Check sheet for the modelled part. Datum: model origin and axes. Units: mm. A direction names the side the tool comes from. Round coordinates to 2 decimals unless told otherwise and drop trailing zeros. Loops run counter-clockwise (first coordinate to the right, second up) from the corner with the lowest first, then second, coordinate; pieces in that order, holes last. Notation, with made-up numbers: (53.5, -26.5) - (62.5, -26.5) arc R11 cw to (62.5, -5.5) - close; hole circle Ø9 at (3, -30.75). An arc over 180 degrees is marked (long way). Put each result on its own line as item: value. Start each with the question number.
Item 1: Section check A-A, the plane x = 0. Record the cut outline in (y, z), and give its area (3 significant figures).
Item 2: Section check D-D, the plane z = -2.5. Record the cut outline in (x, y), and give its area (3 significant figures).
Item 3: Gauge pin test, flat ends, axial feed: pin 1 Ø3 at (y, z) = (3, -1) entering from +X; pin 2 Ø4 at (x, z) = (-5, -5.5) entering from +Y; pin 3 Ø3 at (y, z) = (3.5, 4) entering from -X; pin 4 Ø3 at (y, z) = (10, 0.5) entering from -X. Record the tip position at first contact, or that the pin passes through.
Item 4: Material ranges on line 1 along X through (y, z) = (4.5, 0); line 2 along Y through (x, z) = (-2.5, -4), recorded low to high.
Item 5: Section check B-B, the plane z = 0. Record the cut outline in (x, y), and give its area (3 significant figures).
Item 6: Draft check along X on faces 5 (the cylindrical face through (-3.32, 6.16, -0.74)), 6 (the cylindrical face through (-6.834, 1.972, -1.517)), 7 (the flat face through (0, 12.148, 4)). Enter one of: pulls with the +X half, pulls with the -X half, needs draft (parallel to the pull), parting line crosses it, or undercut.
Item 7: Section check C-C, the plane y = 1. Record the cut outline in (x, z), and give its area (3 significant figures).
Item 8: Tool access check on faces 1 (the flat face through (2, 0, 3)), 2 (the cylindrical face through (0, 8, -5)), 3 (the flat face through (-4.5, 13.6, -1.709)), 4 (the flat face through (-4.5, 13.6, 1.709)). Record the directions out of +Z, -Z, +X, -X, +Y, -Y that give a thin tool (end or side, any length) a straight path to the whole face; none if there is none.
from build123d import *

# Parameters (mm, degrees)
SKETCH_1_R                   = 7
EXTRUDE_1_DEPTH              = 4
SKETCH_5_R                   = 5
EXTRUDE_2_DEPTH              = 11
HOLE_WIZARD_M8_1_D           = 6.8
HOLE_WIZARD_M8_1_ON_FACE_2_D = 6.8
CUT_EXTRUDE_4_DEPTH          = 21.443853316
CUT_EXTRUDE_4_DEPTH_BACK     = 21.443853316
SKETCH_11_W                  = 5.891851166
SKETCH_11_H                  = 2.9
SKETCH_11_W_2                = 4.303127725
SKETCH_12_R                  = 4.6
CUT_EXTRUDE_5_DEPTH          = 2.85


with BuildPart() as part:
    # 草图1 → 凸台-拉伸1 (new body)
    with BuildSketch(Plane(origin=(0, 0, 0), x_dir=(1, 0, 0), z_dir=(0, 1, 0))):
        with Locations(Location((0, 0, 0), (0, 0, 270))):
            Circle(SKETCH_1_R)
    extrude(amount=EXTRUDE_1_DEPTH)

    # 草图5 → 凸台-拉伸2 (add)
    with BuildSketch(Plane(origin=(0, 4, 0), x_dir=(1, 0, 0), z_dir=(0, 1, 0))):
        with Locations(Location((0, 0, 0), (0, 0, 270))):
            Circle(SKETCH_5_R)
    extrude(amount=EXTRUDE_2_DEPTH)

    # M8 螺纹孔1 (through all)
    with Locations(Plane(origin=(0, 0, 0), x_dir=(0, 0, -1), z_dir=(0, -1, 0))):
        with Locations((0, 0)):
            Hole(HOLE_WIZARD_M8_1_D / 2)

    # M8 螺纹孔1 on face 2 (through all)
    with Locations(Plane.ZX.offset(15)):
        with Locations((0, 0)):
            Hole(HOLE_WIZARD_M8_1_ON_FACE_2_D / 2)

    # 草图11 → 切除-拉伸4 (cut, two sides: drawn at the far end of the back side and taken through both)
    with BuildSketch(Plane(origin=(4.997963928, 0, 0), x_dir=(0, 0, -1), z_dir=(1, 0, 0)).offset(-CUT_EXTRUDE_4_DEPTH_BACK)):
        with Locations((4.654854154, 13.597531036)):
            Rectangle(SKETCH_11_W, SKETCH_11_H)
        with Locations((-3.860492434, 13.597531036)):
            Rectangle(SKETCH_11_W_2, SKETCH_11_H)
    extrude(amount=CUT_EXTRUDE_4_DEPTH + CUT_EXTRUDE_4_DEPTH_BACK, mode=Mode.SUBTRACT)

    # 草图12 → 切除-拉伸5 (cut)
    with BuildSketch(Plane(origin=(0, 15, 0), x_dir=(1, 0, 0), z_dir=(0, 1, 0))):
        Circle(SKETCH_12_R)
    extrude(amount=-CUT_EXTRUDE_5_DEPTH, mode=Mode.SUBTRACT)


solid = part.part
Check result:
1. outline: (0, -7) - (4, -7) - (4, -5) - (12.15, -5) - (12.15, -3.4) - (0, -3.4) - close; (0, 3.4) - (12.15, 3.4) - (12.15, 5) - (4, 5) - (4, 7) - (0, 7) - close
1. area: 54.9 mm²
2. outline: (-6.54, 0) - (-2.3, 0) - (-2.3, 12.15) - (-4.33, 12.15) - (-4.33, 4) - (-6.54, 4) - close; (2.3, 0) - (6.54, 0) - (6.54, 4) - (4.33, 4) - (4.33, 12.15) - (2.3, 12.15) - close
2. area: 66.9 mm²
3. pin 1: x = 7
3. pin 2: y = 4
3. pin 3: x = -6.54
3. pin 4: x = -5
4. line 1: -5 to -3.4, 3.4 to 5
4. line 2: 0 to 12.15
5. outline: (-7, 0) - (-3.4, 0) - (-3.4, 12.15) - (-4.6, 12.15) - (-4.6, 15) - (-5, 15) - (-5, 4) - (-7, 4) - close; (3.4, 0) - (7, 0) - (7, 4) - (5, 4) - (5, 15) - (4.6, 15) - (4.6, 12.15) - (3.4, 12.15) - close
5. area: 57.2 mm²
6. face 5: undercut
6. face 6: parting line crosses it
6. face 7: needs draft
7. outline: circle Ø14 at (0, 0); hole circle Ø6.8 at (0, 0)
7. area: 118 mm²
8. face 1: +Z, -Z, +X, -X, -Y
8. face 2: +Y
8. face 3: -Z, +X, -X, +Y
8. face 4: +Z, +X, -X, +Y
